Here's how the part is built. I have some questions about the finished solid (model axes, mm). A direction names the side the tool comes from. Give positions to 0.01 mm unless a question says otherwise; leave off trailing zeros. Loops run counter-clockwise (first coordinate to the right, second up) from the corner with the lowest first, then second, coordinate; pieces in that order, holes last. Notation, with made-up numbers: (-8.5, -29) -> (46.5, -29) arc R26 ccw to (46.5, -5) -> close; hole circle Ø10 at (11, 22.5). An arc over 180 degrees is marked (long way). Answer in a Markdown table with one row per item. Add a question column.
Item 1: If we section it at B-B (z = -0.5): Write out the boundary of the cut face in (x, y) (3 decimals), then the cut area to 3 significant figures.
Item 2: If we section it at C-C (y = -2): Write out the boundary of the cut face in (x, z), then the cut area to 3 significant figures.
Item 3: If we section it at A-A (y = 13.5): Write out the boundary of the cut face in (x, z) (3 decimals), then the cut area to 3 significant figures.
Item 4: We'd pull the mould along Z, two halves only. Please class faces 1 (the face through (0, 12, -11.5)), 2 (the face through (-0.1, 20.1, -8)), 3 (the face through (-6.5, -4, 0)): released by +Z, released by -Z, zero draft, split by the parting line, or undercut.
Item 5: If I drill on line 1 (X direction, y = -8, z = -8.5); line 2 (X direction, y = 15.5, z = -3) (3 decimals); line 3 (Y direction, x = 4.5, z = 3.25), over which ranges is the centre line in solid material (lowest first)?
Item 6: Which directions (+Z, -Z, +X, -X, +Y, -Y) give clear straight access to the entire face, cutting with the end or side of a thin tool? Please do faces 4 (the face through (0, 10, 3.5)), 5 (the face through (0, 26, -11)), 6 (the face through (0, 12, 11.5)), 7 (the face through (6.5, -4, 0)), 8 (the face through (4, 18, 0)).
Item 7: For P1, Ø1.5, axis at x = 5.5, z = -1, coming from the -Y side; P2, Ø1.8, axis at x = 2.5, z = 1.5, coming from the +Y side; P3, Ø0.5, axis at x = 0, z = 3, coming from the -Y side, each with a flat end and sliding along its axis, tell me the tip position at first contact or that it passes through.
Item 8: If we section it at D-D (x = -2.75): Write out the boundary of the cut face in (y, z).
```python
from build123d import *

# Parameters (mm, degrees)
SKETCH1_W           = 15
SKETCH1_H           = 23
BOSS_EXTRUDE1_DEPTH = 26
SKETCH4_W           = 20
SKETCH4_H           = 8
CUT_EXTRUDE2_DEPTH  = 33.144206321
FILLET1_R           = 7
SKETCH5_W           = 15
SKETCH5_H           = 23
BOSS_EXTRUDE2_DEPTH = 10
SKETCH7_W           = 13
SKETCH7_H           = 12
CUT_EXTRUDE3_DEPTH  = 36.514081714
SKETCH11_W          = 1.15
SKETCH11_H          = 7
CUT_EXTRUDE4_DEPTH  = 16


with BuildPart() as part:
    # Sketch1 → Boss-Extrude1 (new body)
    with BuildSketch(Plane(origin=(0, 0, 0), x_dir=(1, 0, 0), z_dir=(0, 1, 0))):
        Rectangle(SKETCH1_W, SKETCH1_H)
    extrude(amount=BOSS_EXTRUDE1_DEPTH)

    # Sketch4 → Cut-Extrude2 (cut, through all)
    with BuildSketch(Plane(origin=(7.5, 0, 0), x_dir=(0, 0, -1), z_dir=(1, 0, 0))):
        with Locations((0, 22)):
            Rectangle(SKETCH4_W, SKETCH4_H)
    extrude(amount=-CUT_EXTRUDE2_DEPTH, mode=Mode.SUBTRACT)

    # Fillet1
    fillet1_edges = [part.edges().sort_by_distance(p)[0] for p in [
        (0, 18, 10),
        (0, 18, -10),
    ]]
    fillet(fillet1_edges, radius=FILLET1_R)

    # Sketch5 → Boss-Extrude2 (add)
    with BuildSketch(Plane.XZ):
        Rectangle(SKETCH5_W, SKETCH5_H)
    extrude(amount=BOSS_EXTRUDE2_DEPTH)

    # Sketch7 → Cut-Extrude3 (cut, through all)
    with BuildSketch(Plane.XY.offset(11.5)):
        with Locations((0, -4)):
            Rectangle(SKETCH7_W, SKETCH7_H)
    extrude(amount=-CUT_EXTRUDE3_DEPTH, mode=Mode.SUBTRACT)

    # Sketch11 → Cut-Extrude4 (cut)
    with BuildSketch(Plane.XZ.offset(-2)):
        Rectangle(SKETCH11_W, SKETCH11_H)
    extrude(amount=-CUT_EXTRUDE4_DEPTH, mode=Mode.SUBTRACT)


solid = part.part
```
Recorded:
| question | item | result |
|---|---|---|
| 1 | outline | (-7.5, -10) -> (-6.5, -10) -> (-6.5, 2) -> (-0.575, 2) -> (-0.575, 18) -> (-7.5, 18) -> close; (0.575, 2) -> (6.5, 2) -> (6.5, -10) -> (7.5, -10) -> (7.5, 18) -> (0.575, 18) -> close |
| 1 | area | 246 mm^2 |
| 2 | outline | (-7.5, -11.5) -> (-6.5, -11.5) -> (-6.5, 11.5) -> (-7.5, 11.5) -> close; (6.5, -11.5) -> (7.5, -11.5) -> (7.5, 11.5) -> (6.5, 11.5) -> close |
| 2 | area | 46.0 mm^2 |
| 3 | outline | (-7.5, -11.5) -> (7.5, -11.5) -> (7.5, 11.5) -> (-7.5, 11.5) -> close; hole (-0.575, -3.5) -> (0.575, -3.5) -> (0.575, 3.5) -> (-0.575, 3.5) -> close |
| 3 | area | 337 mm^2 |
| 4 | face 1 | released by -Z |
| 4 | face 2 | undercut |
| 4 | face 3 | zero draft |
| 5 | line 1 | x = -7.5 to -6.5, 6.5 to 7.5 |
| 5 | line 2 | x = -7.5 to -0.575, 0.575 to 7.5 |
| 5 | line 3 | y = 2 to 18 |
| 6 | face 4 | -Y |
| 6 | face 5 | +Z, -Z, +X, -X, +Y |
| 6 | face 6 | +Z, +X, -X, +Y, -Y |
| 6 | face 7 | +Z, -Z, -Y |
| 6 | face 8 | +X, -X, +Y |
| 7 | P1 | stops at y = 2 |
| 7 | P2 | stops at y = 18 |
| 7 | P3 | stops at y = 18 |
| 8 | outline | (2, -11.5) -> (26, -11.5) -> (26, -10) -> (25, -10) arc R7 cw to (18, -3) -> (18, 3) arc R7 cw to (25, 10) -> (26, 10) -> (26, 11.5) -> (2, 11.5) -> close |
